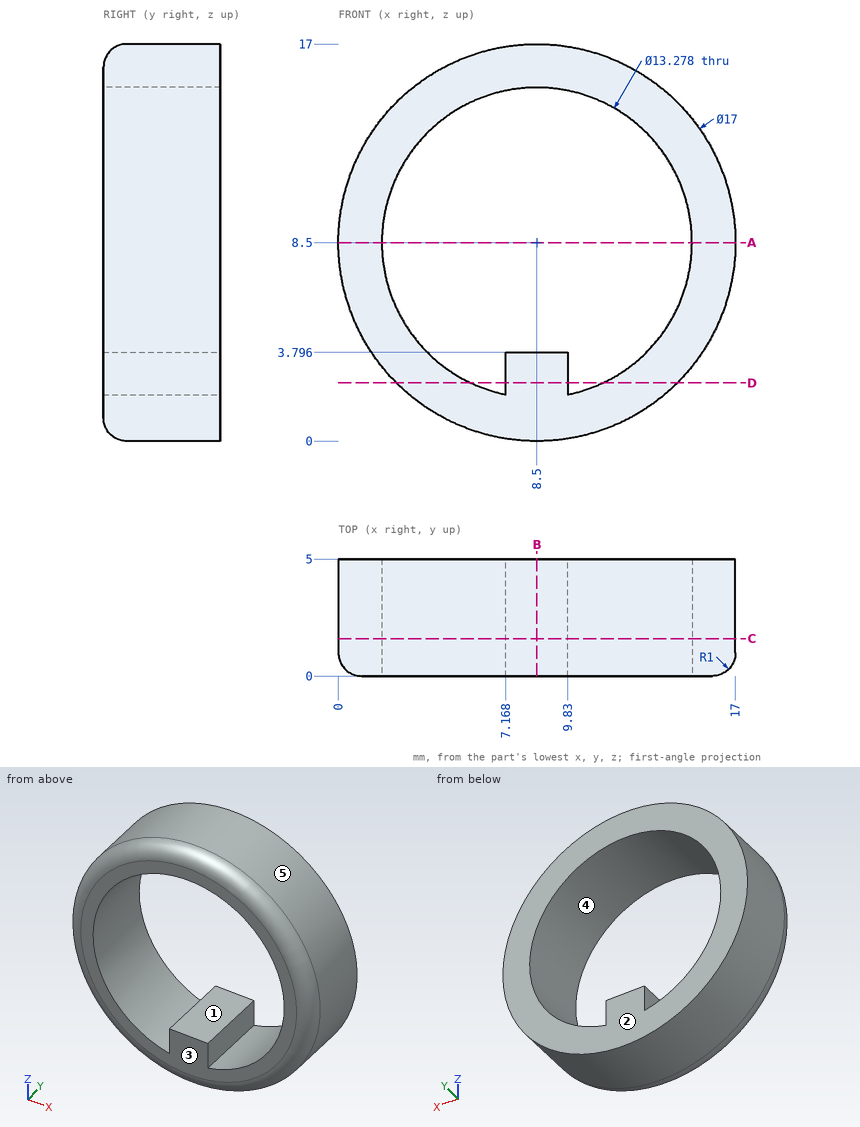
Can you work these out from the drawing? Everything is in mm from the part's minimum corner. A direction names the side the tool comes from. Coordinates: 2 decimals unless noted, no trailing zeros. Loops run counter-clockwise (first coordinate to the right, second up) from the corner with the lowest first, then second, coordinate; pieces in that order, holes last.
1) I need wall thicknesses on probe 1 along Z at (x, y) = (8.5, 3.05); probe 2 along X at (y, z) = (1.15, 8.5); probe 3 along X at (y, z) = (3.55, 10.5). Which ranges of each line are inside material? Lowest first, please.
2) Imagine slicing it at A-A on z = 8.5. List the corners of the cut face in (x, y) for me.
3) For pin 1 (1.4 mm diameter, centred on y = 3.5, z = 3.5, fed in from +X); pin 2 (0.9 mm diameter, centred on y = 3.5, z = 3, fed in from -X); pin 3 (1 mm diameter, centred on x = 8, y = 0.5, fed in from -Z), each with a flat end and sliding along its axis, tell me the tip position at first contact or that it passes through.
4) Imagine slicing it at B-B on x = 8.5. List the corners of the cut face in (y, z) for me.
5) Thinking about a two-plate mould opening in Z: for the marked faces 3, 4 and 5, which applies, pulls with the +Z half, pulls with the -Z half, needs draft (parallel to the pull), parting line crosses it, or undercut?
6) Imagine slicing it at C-C on y = 1.6. List the corners of the cut face in (x, z) for me.
7) Imagine slicing it at D-D on z = 2.5. State how many separate pieces and enclosed holes the cut face has, plus the area to 3 significant figures.
8) Which directions (+Z, -Z, +X, -X, +Y, -Y) give clear straight access to the entire face, cutting with the end or side of a thin tool? Please do the marked faces 1 and 2.
Completed:
1. probe 1: z = 0 to 3.8, 15.14 to 17
1. probe 2: x = 0 to 1.86, 15.14 to 17
1. probe 3: x = 0.24 to 2.17, 14.83 to 16.76
2. outline: (0, 1) arc R1 ccw to (1, 0) - (1.86, 0) - (1.86, 5) - (0, 5) - close; (15.14, 0) - (16, 0) arc R1 ccw to (17, 1) - (17, 5) - (15.14, 5) - close
3. pin 1: stops at x = 15.83
3. pin 2: stops at x = 1.66
3. pin 3: stops at z = 0.01
4. outline: (0, 1) arc R1 ccw to (1, 0) - (5, 0) - (5, 3.8) - (0, 3.8) - close; (0, 15.14) - (5, 15.14) - (5, 17) - (1, 17) arc R1 ccw to (0, 16) - close
5. face 3: needs draft
5. face 4: undercut
5. face 5: parting line crosses it
6. outline: circle Ø17 at (8.5, 8.5); hole (7.17, 2) - (7.17, 3.8) - (9.83, 3.8) - (9.83, 2) arc R6.64 ccw (long way) to start
7. separate pieces: 3
7. enclosed holes: 0
7. area: 44.5 mm2
8. face 1: +Y, -Y
8. face 2: +Z, -Z, +X, -X, +Y
